from build123d import *

# Parameters (mm, degrees)
F0_R     = 4.425
F1_DEPTH = 2
F0_R_2   = 6.425
F2_DEPTH = 7
F3_DEPTH = 4.15


with BuildPart() as f1:
    # F0 (on Top) → F1 (new body)
    with BuildSketch(Plane.XY):
        Circle(F0_R)
        Polygon((1.816103, -1.068927), (-0.017667, -2.107254), (-1.833769, -1.038327), (-1.816103, 1.068927), (0.017667, 2.107254), (1.833769, 1.038327), align=None, mode=Mode.SUBTRACT)
    extrude(amount=F1_DEPTH)

    # F0 (on Top) → F2 (join)
    with BuildSketch(Plane.XY):
        Circle(F0_R_2)
        Circle(F0_R, mode=Mode.SUBTRACT)
    extrude(amount=F2_DEPTH)

    # F0 (on Top) → F3 (join)
    with BuildSketch(Plane.XY):
        Polygon((-1.833769, -1.038327), (-0.017667, -2.107254), (1.816103, -1.068927), (1.833769, 1.038327), (0.017667, 2.107254), (-1.816103, 1.068927), align=None)
    extrude(amount=F3_DEPTH)


solid = f1.part
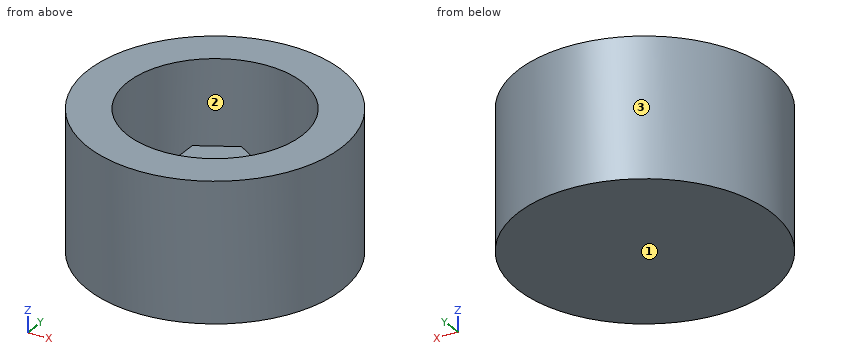
Build history of the part. All positions in model axes, mm. Face numbers are marked on the shaded views. Give positions to 0.01 mm unless a question says otherwise; leave off trailing zeros. Loops run counter-clockwise (first coordinate to the right, second up) from the corner with the lowest first, then second, coordinate; pieces in that order, holes last. Notation, with made-up numbers: (61.5, 57.25) -> (77.5, 57.25) arc R27 cw to (77.5, 93.25) -> close; hole circle Ø9 at (-13.75, 70.5). An arc over 180 degrees is marked (long way). Answer in a Markdown table with one row per item.
Item 1: Probe line 1 along Y through (x, z) = (-1.25, 3.5); line 2 along Y through (x, z) = (0, 5.25) (3 decimals); line 3 along Y through (x, z) = (0, 3.95) (3 decimals). List the from-to ranges inside material, lowest first. Write a range as [from, to].
Findings below:
| item | result |
|---|---|
| line 1 | y = [-6.3, -4.24], [-1.38, 1.39], [4.24, 6.3] |
| line 2 | y = [-6.425, -4.425], [4.425, 6.425] |
| line 3 | y = [-6.425, -4.425], [-2.097, 2.097], [4.425, 6.425] |
Item 2: Flat gauge pins, fed straight in: P1, Ø1, axis at y = 1, z = 2.5, coming from the +X side; P2, Ø4.5, axis at x = 1.5, y = -0.5, coming from the +Z side; P3, Ø1.5, axis at y = 4, z = 5.5, coming from the -X side. Where does each tip first touch, or does it go through?
Findings below:
| item | result |
|---|---|
| P1 | stops at x = 6.41 |
| P2 | stops at z = 4.15 |
| P3 | stops at x = -5.54 |
Item 3: Slice it at C-C on z = 4.5. Write the cut outline in (x, y) (3 decimals).
Findings below:
| item | result |
|---|---|
| outline | circle Ø12.85 at (0, 0); hole circle Ø8.85 at (0, 0) |
Item 4: Mould opens along X. For the marked faces 1, 2 and 3 say: pulls with the +X half, pulls with the -X half, needs draft (parallel to the pull), parting line crosses it, or undercut.
Findings below:
| item | result |
|---|---|
| face 1 | needs draft |
| face 2 | undercut |
| face 3 | parting line crosses it |
Item 5: Slice it at B-B on y = 0.25. Write the cut outline in (x, z).
Findings below:
| item | result |
|---|---|
| outline | (-6.42, 0) -> (6.42, 0) -> (6.42, 7) -> (4.42, 7) -> (4.42, 2) -> (1.83, 2) -> (1.83, 4.15) -> (-1.82, 4.15) -> (-1.82, 2) -> (-4.42, 2) -> (-4.42, 7) -> (-6.42, 7) -> close |
Item 6: Slice it at D-D on z = 0.5. Write the cut outline in (x, y) (3 decimals), plus the area to 3 significant figures.
Findings below:
| item | result |
|---|---|
| outline | circle Ø12.85 at (0, 0) |
| area | 130 mm² |
Item 7: Slice it at A-A on x = 1.25. Write the cut outline in (y, z).
Findings below:
| item | result |
|---|---|
| outline | (-6.3, 0) -> (6.3, 0) -> (6.3, 7) -> (4.24, 7) -> (4.24, 2) -> (1.38, 2) -> (1.38, 4.15) -> (-1.39, 4.15) -> (-1.39, 2) -> (-4.24, 2) -> (-4.24, 7) -> (-6.3, 7) -> close |
